from build123d import *

# Parameters (mm, degrees)
F0_W     = 76.2
F0_H     = 15.875
F1_DEPTH = 0.79375
F2_R     = 1.7859375
F3_DEPTH = 1.5875
F4_W     = 76.2
F4_H     = 1.5875
F5_DEPTH = 14.2875
F6_R     = 1.7859375
F6_R_2   = 1.7907
F7_DEPTH = 1.5875


# Not quite as in the source:
# - a pattern or mirror of a feature is missing from the dataset's text; its kind, count and spacing are read off the source's solid


with BuildPart() as f1:
    # F0 (on Front) → F1 (new body, symmetric)
    with BuildSketch(Plane.XZ):
        Rectangle(F0_W, F0_H)
    extrude(amount=F1_DEPTH, both=True)

    # F2 (on face) → F3 (cut, through all)
    with BuildSketch(Plane.XZ.offset(0.79375)):
        with Locations((-25.4, 0)):
            Circle(F2_R)
    f3 = extrude(amount=-F3_DEPTH, mode=Mode.SUBTRACT)

    # F3_copies: F3 across plane
    add(f3.mirror(Plane(origin=(0, 0, 0), x_dir=(0, 0, 1), z_dir=(1, 0, 0))), mode=Mode.SUBTRACT)

    # F4 (on face) → F5 (join)
    with BuildSketch(Plane.XZ.offset(0.79375)):
        with Locations((0, -7.14375)):
            Rectangle(F4_W, F4_H)
    extrude(amount=F5_DEPTH)

    # F6 (on face) → F7 (cut, through all)
    with BuildSketch(Plane.XY.offset(-6.35)):
        with Locations((-19.05, -7.14375)):
            Circle(F6_R)
        with Locations((19.05, -7.14375)):
            Circle(F6_R_2)
    extrude(amount=-F7_DEPTH, mode=Mode.SUBTRACT)


solid = f1.part
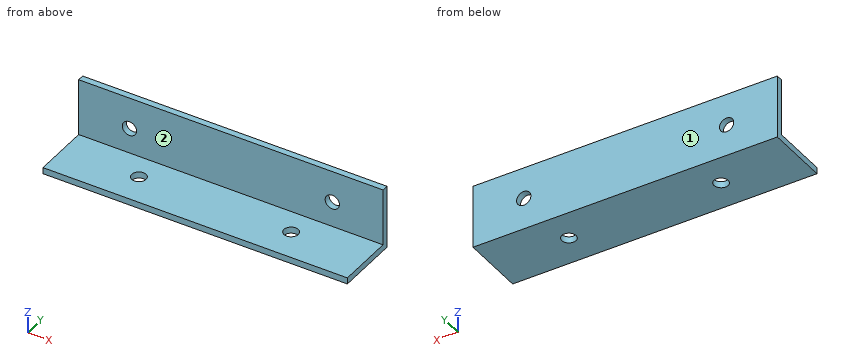
Can you work these out from the model? Positions are in its coordinate system, mm. Face numbers are marked on the shaded views. A direction names the side the tool comes from. Give positions to 0.01 mm unless a question says otherwise; leave off trailing zeros. Loops run counter-clockwise (first coordinate to the right, second up) from the corner with the lowest first, then second, coordinate; pieces in that order, holes last. Notation, with made-up numbers: (13, 83.25) -> (49, 83.25) arc R23 cw to (49, 95.25) -> close; hole circle Ø6 at (35.25, -39). An arc over 180 degrees is marked (long way). Return JSON: item names as keys, results as strings.
Q1. I want a section at D-D, the plane x = -4. List the corners of the cut face in (y, z) for me, then the cut area to 3 significant figures.
Checks:
{"outline": "(-15.08, -7.94) -> (0.79, -7.94) -> (0.79, 7.94) -> (-0.79, 7.94) -> (-0.79, -6.35) -> (-15.08, -6.35) -> close", "area": "47.9 mm2"}
Q2. I want a section at C-C, the plane y = -6. List the corners of the cut face in (x, z) for me.
Checks:
{"outline": "(-38.1, -7.94) -> (-20.42, -7.94) -> (-20.42, -6.35) -> (-38.1, -6.35) -> close; (-17.68, -7.94) -> (17.67, -7.94) -> (17.67, -6.35) -> (-17.68, -6.35) -> close; (20.43, -7.94) -> (38.1, -7.94) -> (38.1, -6.35) -> (20.43, -6.35) -> close"}
Q3. I want a section at A-A, the plane x = 19.05. List the corners of the cut face in (y, z) for me.
Checks:
{"outline": "(-15.08, -7.94) -> (-8.93, -7.94) -> (-8.93, -6.35) -> (-15.08, -6.35) -> close; (-5.35, -7.94) -> (0.79, -7.94) -> (0.79, 7.94) -> (-0.79, 7.94) -> (-0.79, -6.35) -> (-5.35, -6.35) -> close"}
Q4. On a 3-axis mill with a long thin cutter (end or side, diameter ignored), from which of +Z, -Z, +X, -X, +Y, -Y can I reach the whole of each face in a straight line? I mean the marked faces 1 and 2. Say none if no direction works.
Checks:
{"face 1": "+Z, -Z, +X, -X, +Y", "face 2": "+Z, +X, -X, -Y"}
Q5. I need wall thicknesses on probe 1 along Z at (x, y) = (25.4, 0.3); probe 2 along Y at (x, z) = (20.5, -1.25); probe 3 along Z at (x, y) = (-1, -5.25). Which ranges of each line are inside material? Lowest first, please.
Checks:
{"probe 1": "z = -7.94 to -1.79, 1.79 to 7.94", "probe 2": "y = -0.79 to 0.79", "probe 3": "z = -7.94 to -6.35"}
Q6. For pin 1 Ø5 at (x, z) = (7, -6) entering from -Y; pin 2 Ø3 at (x, z) = (25.4, 0) entering from +Y; pin 3 Ø1 at (x, y) = (25.5, -8) entering from +Z; pin 4 Ø4.5 at (x, z) = (15.5, 2.5) entering from -Y, each with a flat end and sliding along its axis, tell me the tip position at first contact or that it passes through.
Checks:
{"pin 1": "stops at y = -15.08", "pin 2": "passes through", "pin 3": "stops at z = -6.35", "pin 4": "stops at y = -0.79"}
Q7. I want a section at B-B, the plane z = 0. List the corners of the cut face in (x, y) for me.
Checks:
{"outline": "(-38.1, -0.79) -> (-27.19, -0.79) -> (-27.19, 0.79) -> (-38.1, 0.79) -> close; (-23.61, -0.79) -> (23.61, -0.79) -> (23.61, 0.79) -> (-23.61, 0.79) -> close; (27.19, -0.79) -> (38.1, -0.79) -> (38.1, 0.79) -> (27.19, 0.79) -> close"}
